Design review of the part built by this model. Coordinates are the model's own, in mm. Give positions to 0.01 mm unless a question says otherwise; leave off trailing zeros. Loops run counter-clockwise (first coordinate to the right, second up) from the corner with the lowest first, then second, coordinate; pieces in that order, holes last. Notation, with made-up numbers: (13.25, 39) -> (17.25, 39) arc R26 cw to (17.25, 77) -> close; hole circle Ø10 at (58, 40.5). An arc over 180 degrees is marked (long way). Answer in a Markdown table with one row per item. Add a question column.
(1) Consider section B-B on z = 7. Write out the cut boundary in (x, y), then the cut area to 3 significant figures.
(2) For pin 1 (2 mm diameter, centred on x = 28.5, z = 21.5, fed in from -Y); pin 2 (5.5 mm diameter, centred on x = 46, y = 2, fed in from -Z), all flat-tipped, find the tip position at first contact; note any pin that passes through.
(3) For line 1 (Z direction, x = 17, y = 7.5); line 2 (Z direction, x = 35, y = 8.7); line 3 (Y direction, x = -43.85, z = -28.5), list the stretches that pass through material, from the lowest coordinate up.
(4) Consider section A-A on x = -17.5. Write out the cut boundary in (y, z), then the cut area to 3 significant figures.
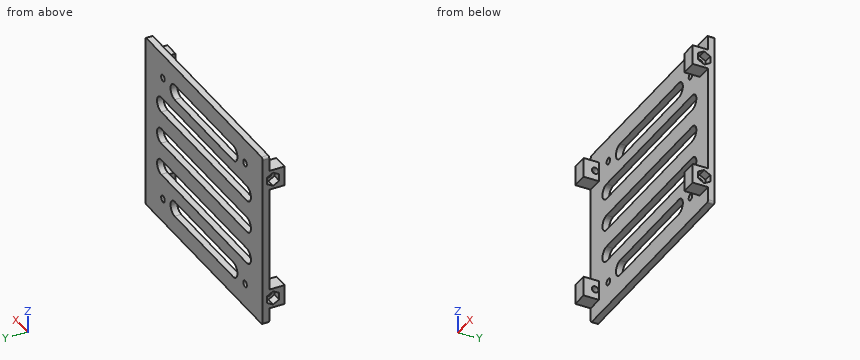
from build123d import *

# Parameters (mm, degrees)
EXTRUDE_1_DEPTH                            = 10
CUT_EXTRUDE_1_DEPTH                        = 7
CUT_EXTRUDE_3_DEPTH                        = 4
CUT_EXTRUDE_4_DEPTH                        = 65.412731661
CUT_EXTRUDE_6_REACH                        = 106.48
SKETCH_8_R                                 = 1.5
CUT_EXTRUDE_6_DIRECTION_2_DEPTH            = 105.479663093
MIRROR_2_AT_THE_SECOND_PLANE_COPY_1_REACH  = 106.48
MIRROR_2_AT_THE_SECOND_PLANE_COPY_1_SKET_R = 1.5
MIRROR_2_AT_THE_SECOND_PLANE_COPY_2_SKET_R = 1.5
MIRROR_2_AT_THE_SECOND_PLANE_COPY_2_DEPTH  = 105.479663093
MIRROR_2_AT_THE_SECOND_PLANE_COPY_3_SKET_R = 1.5
MIRROR_2_AT_THE_SECOND_PLANE_COPY_3_DEPTH  = 105.479663093
CUT_EXTRUDE_7_REACH                        = 66.413
SKETCH_9_R                                 = 1.5
MIRROR_3_AT_THE_SECOND_PLANE_COPY_1_REACH  = 66.413
MIRROR_3_AT_THE_SECOND_PLANE_COPY_1_SKET_R = 1.5


with BuildPart() as part:
    # 草图1 → 凸台-拉伸1 (new body)
    with BuildSketch(Plane(origin=(0, 0, 0), x_dir=(1, 0, 0), z_dir=(0, 1, 0))):
        with BuildLine():
            Line((-49, 40), (49, 40))
            ThreePointArc((49, 40), (49.707106781, 39.707106781), (50, 39))
            Line((50, 39), (50, -39))
            ThreePointArc((50, -39), (49.707106781, -39.707106781), (49, -40))
            Line((49, -40), (-49, -40))
            ThreePointArc((-49, -40), (-49.707106781, -39.707106781), (-50, -39))
            Line((-50, -39), (-50, 39))
            ThreePointArc((-50, 39), (-49.707106781, 39.707106781), (-49, 40))
        make_face()
    extrude(amount=EXTRUDE_1_DEPTH)

    # 草图2 → 切除-拉伸1 (cut)
    with BuildSketch(Plane(origin=(0, 0, 0), x_dir=(-1, 0, 0), z_dir=(0, -1, 0))):
        Polygon((-50, 33), (-43, 33), (-43, 24), (-50, 24), (-50, -24), (-43, -24), (-43, -33), (-50, -33), (-50, -40), (50, -40), (50, -33), (43, -33), (43, -24), (50, -24), (50, 24), (43, 24), (43, 33), (50, 33), (50, 40), (-50, 40), align=None)
    extrude(amount=-CUT_EXTRUDE_1_DEPTH, mode=Mode.SUBTRACT)

    # 草图5 → 切除-拉伸3 (cut)
    with BuildSketch(Plane.ZY.offset(50)):
        Polygon((30.08771324, 7.998490707), (31.675426481, 5.248490707), (30.08771324, 2.498490707), (26.91228676, 2.498490707), (25.324573519, 5.248490707), (26.91228676, 7.998490707), align=None)
        Polygon((-25.324573519, 5.248490707), (-26.91228676, 7.998490707), (-30.08771324, 7.998490707), (-31.675426481, 5.248490707), (-30.08771324, 2.498490707), (-26.91228676, 2.498490707), align=None)
    cut_extrude_3 = extrude(amount=-CUT_EXTRUDE_3_DEPTH, mode=Mode.SUBTRACT)

    # 镜向1: 切除-拉伸3 across plane
    add(cut_extrude_3.mirror(Plane(origin=(0, 0, 0), x_dir=(0, 0, 1), z_dir=(1, 0, 0))), mode=Mode.SUBTRACT)

    # 草图6 → 切除-拉伸4 (cut, through all)
    with BuildSketch(Plane(origin=(0, 7, 0), x_dir=(-1, 0, 0), z_dir=(0, -1, 0))):
        with BuildLine():
            Line((25, -31.5), (-25, -31.5))
            ThreePointArc((-25, -31.5), (-28.5, -28), (-25, -24.5))
            Line((-25, -24.5), (25, -24.5))
            ThreePointArc((25, -24.5), (28.5, -28), (25, -31.5))
        make_face()
        with BuildLine():
            Line((25, 31.5), (-25, 31.5))
            ThreePointArc((-25, 31.5), (-28.5, 28), (-25, 24.5))
            Line((-25, 24.5), (25, 24.5))
            ThreePointArc((25, 24.5), (28.5, 28), (25, 31.5))
        make_face()
        with BuildLine():
            Line((-36.5, -11.876137074), (36.5, -11.876137074))
            ThreePointArc((36.5, -11.876137074), (40, -15.376137074), (36.5, -18.876137074))
            Line((36.5, -18.876137074), (-36.5, -18.876137074))
            ThreePointArc((-36.5, -18.876137074), (-40, -15.376137074), (-36.5, -11.876137074))
        make_face()
        with BuildLine():
            Line((-36.5, 3.123862926), (36.5, 3.123862926))
            ThreePointArc((36.5, 3.123862926), (40, -0.376137074), (36.5, -3.876137074))
            Line((36.5, -3.876137074), (-36.5, -3.876137074))
            ThreePointArc((-36.5, -3.876137074), (-40, -0.376137074), (-36.5, 3.123862926))
        make_face()
        with BuildLine():
            Line((-36.5, 18.123862926), (36.5, 18.123862926))
            ThreePointArc((36.5, 18.123862926), (40, 14.623862926), (36.5, 11.123862926))
            Line((36.5, 11.123862926), (-36.5, 11.123862926))
            ThreePointArc((-36.5, 11.123862926), (-40, 14.623862926), (-36.5, 18.123862926))
        make_face()
    extrude(amount=-CUT_EXTRUDE_4_DEPTH, mode=Mode.SUBTRACT)

    # 草图8 → 切除-拉伸6 (cut, up to next)
    with BuildSketch(Plane.ZY.offset(46), mode=Mode.PRIVATE) as cut_extrude_6_sk1:
        with Locations((-28.5, 5.248490707)):
            Circle(SKETCH_8_R)
    cut_extrude_6_tool1 = extrude(cut_extrude_6_sk1.sketch, amount=-CUT_EXTRUDE_6_REACH, mode=Mode.PRIVATE) & part.part
    cut_extrude_6 = cut_extrude_6_tool1.solids().sort_by_distance((-46, 5.248491, -28.5))[0]
    add(cut_extrude_6, mode=Mode.SUBTRACT)

    # 草图8 → 切除-拉伸6 direction 2 (cut)
    with BuildSketch(Plane.ZY.offset(46)):
        with Locations((-28.5, 5.248490707)):
            Circle(SKETCH_8_R)
    cut_extrude_6_direction_2 = extrude(amount=CUT_EXTRUDE_6_DIRECTION_2_DEPTH, mode=Mode.SUBTRACT)

    # 镜向2: 切除-拉伸6, 切除-拉伸6 direction 2 across plane
    add(cut_extrude_6.mirror(Plane(origin=(0, 0, 0), x_dir=(0, 0, 1), z_dir=(1, 0, 0))), mode=Mode.SUBTRACT)
    add(cut_extrude_6_direction_2.mirror(Plane(origin=(0, 0, 0), x_dir=(0, 0, 1), z_dir=(1, 0, 0))), mode=Mode.SUBTRACT)

    # 镜向2 at the second plane: 切除-拉伸6, 切除-拉伸6 direction 2 across plane
    add(cut_extrude_6.mirror(Plane.XY), mode=Mode.SUBTRACT)
    add(cut_extrude_6_direction_2.mirror(Plane.XY), mode=Mode.SUBTRACT)

    # 镜向2 at the second plane copy 1 sket → 镜向2 at the second plane copy 1 (cut, up to next)
    with BuildSketch(Plane(origin=(46, 0, 0), x_dir=(0, 0, -1), z_dir=(1, 0, 0)), mode=Mode.PRIVATE) as mirror_2_at_the_second_plane_copy_1_sk1:
        with Locations((-28.5, 5.248490707)):
            Circle(MIRROR_2_AT_THE_SECOND_PLANE_COPY_1_SKET_R)
    mirror_2_at_the_second_plane_copy_1_tool1 = extrude(mirror_2_at_the_second_plane_copy_1_sk1.sketch, amount=-MIRROR_2_AT_THE_SECOND_PLANE_COPY_1_REACH, mode=Mode.PRIVATE) & part.part
    add(mirror_2_at_the_second_plane_copy_1_tool1.solids().sort_by_distance((46, 5.248491, 28.5))[0], mode=Mode.SUBTRACT)

    # 镜向2 at the second plane copy 2 sket → 镜向2 at the second plane copy 2 (cut)
    with BuildSketch(Plane(origin=(46, 0, 0), x_dir=(0, 0, -1), z_dir=(1, 0, 0))):
        with Locations((-28.5, 5.248490707)):
            Circle(MIRROR_2_AT_THE_SECOND_PLANE_COPY_2_SKET_R)
    extrude(amount=MIRROR_2_AT_THE_SECOND_PLANE_COPY_2_DEPTH, mode=Mode.SUBTRACT)

    # 镜向2 at the second plane copy 3 sket → 镜向2 at the second plane copy 3 (cut)
    with BuildSketch(Plane(origin=(-46, 0, 0), x_dir=(0, 0, -1), z_dir=(-1, 0, 0))):
        with Locations((-28.5, -5.248490707)):
            Circle(MIRROR_2_AT_THE_SECOND_PLANE_COPY_3_SKET_R)
    extrude(amount=MIRROR_2_AT_THE_SECOND_PLANE_COPY_3_DEPTH, mode=Mode.SUBTRACT)

    # 草图9 → 切除-拉伸7 (cut, up to next)
    with BuildSketch(Plane(origin=(0, 7, 0), x_dir=(-1, 0, 0), z_dir=(0, -1, 0)), mode=Mode.PRIVATE) as cut_extrude_7_sk1:
        with Locations(Location((35, -29, 0), (0, 0, 90))):
            Circle(SKETCH_9_R)
    cut_extrude_7_tool1 = extrude(cut_extrude_7_sk1.sketch, amount=-CUT_EXTRUDE_7_REACH, mode=Mode.PRIVATE) & part.part
    cut_extrude_7 = cut_extrude_7_tool1.solids().sort_by_distance((-35, 7, 29))[0]
    add(cut_extrude_7, mode=Mode.SUBTRACT)

    # 镜向3: 切除-拉伸7 across plane
    add(cut_extrude_7.mirror(Plane.XY), mode=Mode.SUBTRACT)

    # 镜向3 at the second plane: 切除-拉伸7 across plane
    add(cut_extrude_7.mirror(Plane(origin=(0, 0, 0), x_dir=(0, 0, 1), z_dir=(1, 0, 0))), mode=Mode.SUBTRACT)

    # 镜向3 at the second plane copy 1 sket → 镜向3 at the second plane copy 1 (cut, up to next)
    with BuildSketch(Plane.XZ.offset(-7), mode=Mode.PRIVATE) as mirror_3_at_the_second_plane_copy_1_sk1:
        with Locations(Location((35, -29, 0), (0, 0, 90))):
            Circle(MIRROR_3_AT_THE_SECOND_PLANE_COPY_1_SKET_R)
    mirror_3_at_the_second_plane_copy_1_tool1 = extrude(mirror_3_at_the_second_plane_copy_1_sk1.sketch, amount=-MIRROR_3_AT_THE_SECOND_PLANE_COPY_1_REACH, mode=Mode.PRIVATE) & part.part
    add(mirror_3_at_the_second_plane_copy_1_tool1.solids().sort_by_distance((35, 7, -29))[0], mode=Mode.SUBTRACT)


solid = part.part
Values follow:
| question | item | result |
|---|---|---|
| 1 | outline | (-50, 7) -> (50, 7) -> (50, 10) -> (-50, 10) -> close |
| 1 | area | 300 mm2 |
| 2 | pin 1 | y = 7 |
| 2 | pin 2 | z = -33 |
| 3 | line 1 | -40 to -31.5, -24.5 to -18.12, -11.12 to -3.12, 3.88 to 11.88, 18.88 to 24.5, 31.5 to 40 |
| 3 | line 2 | -40 to -30.5, -27.5 to -18.12, -11.12 to -3.12, 3.88 to 11.88, 18.88 to 27.5, 30.5 to 40 |
| 3 | line 3 | 0 to 3.75, 6.75 to 10 |
| 4 | outline | (7, -40) -> (10, -40) -> (10, -31.5) -> (7, -31.5) -> close; (7, -24.5) -> (10, -24.5) -> (10, -18.12) -> (7, -18.12) -> close; (7, -11.12) -> (10, -11.12) -> (10, -3.12) -> (7, -3.12) -> close; (7, 3.88) -> (10, 3.88) -> (10, 11.88) -> (7, 11.88) -> close; (7, 18.88) -> (10, 18.88) -> (10, 24.5) -> (7, 24.5) -> close; (7, 31.5) -> (10, 31.5) -> (10, 40) -> (7, 40) -> close |
| 4 | area | 135 mm2 |
